from build123d import *

# Parameters (mm, degrees)
CUT_EXTRUDE_START   = -8.5
CUT_EXTRUDE_5_DEPTH = 8.5
CHAMFER_2_SIZE      = 0.8


with BuildPart() as part:
    # Sketch 16 → Revolve 1 (revolve)
    with BuildSketch(Plane(origin=(0, 0, 0), x_dir=(0, 0, -1), z_dir=(1, 0, 0)), mode=Mode.PRIVATE) as revolve_1_sk:
        Polygon((-45, 0), (-45, 8), (-18.4, 8), (-18.4, 6.4), (-17, 6.4), (-17, 8.6), (-16.3, 9.3), (-4.95, 9.3), (-4.25, 10), (0, 10), (400, 10), (400, 0), align=None)
    revolve(revolve_1_sk.sketch.rotate(Axis((0, 0, -400), (0, 0, 1)), 90), axis=Axis((0, 0, -400), (0, 0, 1)))

    # Sketch 17 → Cut-Extrude 5 (cut)
    with BuildSketch(Plane.XY.offset(17).offset(CUT_EXTRUDE_START)):
        with BuildLine():
            Line((8.2, 4.387482194), (8.2, -4.387482194))
            ThreePointArc((8.2, -4.387482194), (9.3, 0), (8.2, 4.387482194))
        make_face()
        with BuildLine():
            Line((-8.2, 4.387482194), (-8.2, -4.387482194))
            ThreePointArc((-8.2, -4.387482194), (-9.3, 0), (-8.2, 4.387482194))
        make_face()
    extrude(amount=CUT_EXTRUDE_5_DEPTH, mode=Mode.SUBTRACT)

    # Chamfer 2
    chamfer_2_edges = [part.edges().sort_by_distance(p)[0] for p in [
        (8, 0, 45),
    ]]
    chamfer(chamfer_2_edges, length=CHAMFER_2_SIZE)


solid = part.part
Can you work these out from the model? Positions are in its coordinate system, mm. A direction names the side the tool comes from. Coordinates: 2 decimals unless noted, no trailing zeros. Loops run counter-clockwise (first coordinate to the right, second up) from the corner with the lowest first, then second, coordinate; pieces in that order, holes last. Notation, with made-up numbers: (-16.75, 79.5) - (26.25, 79.5) arc R25 ccw to (26.25, 118.5) - close; hole circle Ø2 at (56.5, 44.25). An arc over 180 degrees is marked (long way). Answer as a JSON object with one key per item and string values. Group by question number.
Item 1: On a 3-axis mill with a long thin cutter (end or side, diameter ignored), from which of +Z, -Z, +X, -X, +Y, -Y can I reach the whole of each face in a straight line? I mean faces 5 (the face through (-8.2, 0, 13)), 6 (the face through (-6.104, -1.922, 17.69)), 7 (the face through (6.85, -6.29, 10.55)). Say none if no direction works.
Item 2: If we section it at A-A (x = 0): List the corners of the cut face in (y, z) for me, plus the area to 3 significant figures.
Item 3: If we section it at B-B (z = -40.5): List the corners of the cut face in (x, y) for me, plus the area to 3 significant figures.
Item 4: For pin 1 (9.5 mm diameter, centred on y = 0, z = 10.5, fed in from +X); pin 2 (4 mm diameter, centred on y = -4, z = -218.5, fed in from -X); pin 3 (3 mm diameter, centred on y = -6, z = -200, fed in from -X), each with a flat end and sliding along its axis, tell me the tip position at first contact or that it passes through.
Item 5: If I drill on L1, parallel to Z at x = -4.5, y = 5.25; L2, parallel to X at y = -0.25, z = -282.5; L3, parallel to X at y = 5.75, z = -169, over which ranges is the centre line in solid material (lowest first)? Write a range as from..to.
Item 6: If we mould it in two halves opening along Z, with no side actions, what happens to faces 1 (the face through (0, -7, 18.4)), 2 (the face through (8.2, 0, 13)), 3 (the face through (0, 0, 45)), 4 (the face through (4, 6, 17))? For each: released by +Z, released by -Z, zero draft, split by the parting line, or undercut.
Returned:
{
 "1": {"face 5": "+Z, -X, +Y, -Y", "face 6": "none", "face 7": "+Z"},
 "2": {"outline": "(-10, -400) - (10, -400) - (10, 4.25) - (9.3, 4.95) - (9.3, 16.3) - (8.6, 17) - (6.4, 17) - (6.4, 18.4) - (8, 18.4) - (8, 44.2) - (7.2, 45) - (-7.2, 45) - (-8, 44.2) - (-8, 18.4) - (-6.4, 18.4) - (-6.4, 17) - (-8.6, 17) - (-9.3, 16.3) - (-9.3, 4.95) - (-10, 4.25) - close", "area": "8,770 mm²"},
 "3": {"outline": "circle Ø20 at (0, 0)", "area": "314 mm²"},
 "4": {"pin 1": "stops at x = 9.3", "pin 2": "stops at x = -9.8", "pin 3": "stops at x = -8.93"},
 "5": {"L1": "z = -400..17, 18.4..45", "L2": "x = -10..10", "L3": "x = -8.18..8.18"},
 "6": {"face 1": "undercut", "face 2": "zero draft", "face 3": "released by +Z", "face 4": "undercut"}
}
